```python
from build123d import *


with BuildPart() as part:
    # Sketch1 → Revolve2 (revolve)
    with BuildSketch(Plane.XY):
        with BuildLine():
            Line((-50.8, 69.85), (-50.8, 82.55))
            Line((-50.8, 82.55), (101.6, 82.55))
            Line((101.6, 82.55), (101.6, 12.7))
            Line((101.6, 12.7), (0, 12.7))
            Line((0, 12.7), (0, 25.4))
            ThreePointArc((0, 25.4), (-2.025659238, 31.58997261), (-7.62, 34.925))
            Line((-7.62, 34.925), (-24.13, 34.925))
            ThreePointArc((-24.13, 34.925), (-29.664711714, 38.307730629), (-31.75, 44.45))
            Line((-31.75, 44.45), (-31.75, 57.15))
            ThreePointArc((-31.75, 57.15), (-35.469743879, 66.130256121), (-44.45, 69.85))
            Line((-44.45, 69.85), (-50.8, 69.85))
        make_face()
    revolve(axis=Axis((0, 0, 0), (1, 0, 0)))


solid = part.part
```
The model under review builds one solid part; all positions refer to its coordinate system, in mm. A direction names the side the tool comes from. Round coordinates to 2 decimals unless told otherwise and drop trailing zeros. Loops run counter-clockwise (first coordinate to the right, second up) from the corner with the lowest first, then second, coordinate; pieces in that order, holes last. Notation, with made-up numbers: (-32.5, 9) -> (20.5, 9) arc R24 cw to (20.5, 47) -> close; hole circle Ø2 at (33, -19.75). An arc over 180 degrees is marked (long way). Answer as a JSON object with one key per item and string values. Group by question number.
1) Mouldability with a two-part tool opening along Y and no side actions: class faces 1 (the face through (26.467, -17.895, -80.587)), 2 (the face through (-47.669, -55.431, -42.503)), 3 (the face through (101.6, -1, -17)) as released by +Y, released by -Y, zero draft, split by the parting line, or undercut.
2) For pin 1 Ø5 at (x, y) = (60, -28.5) entering from -Z; pin 2 Ø4 at (x, z) = (26, -32) entering from -Y; pin 3 Ø3 at (y, z) = (63, 1.5) entering from -X; pin 4 Ø15 at (y, z) = (0, 0) entering from +X, all flat-tipped, find the tip position at first contact; note any pin that passes through.
3) We need section C-C on x = 18.5. Write out the cut boundary in (y, z), then the cut area to 3 significant figures.
4) For line 1 (Z direction, x = 60, y = 0); line 2 (Z direction, x = -47, y = 0); line 3 (X direction, y = 15, z = -10.5), list the stretches that pass through material, from the lowest coordinate up. Write a range as [from, to].
5) We need section A-A on z = 0. Write out the cut boundary in (x, y) (3 decimals), then the cut area to 3 significant figures.
6) For faces 4 (the face through (0, -5, 12)), 5 (the face through (50.09, -2.75, -12.4)), list the 3-axis set-ups (+Z, -Z, +X, -X, +Y, -Y) from which the entire face can be reached by the end or side of a thin tool; tool diameter is ignored.
7) We need section D-D on x = -39.5. Write out the cut boundary in (y, z), then the cut area to 3 significant figures.
Result set:
{
 "1": {"face 1": "split by the parting line", "face 2": "undercut", "face 3": "zero draft"},
 "2": {"pin 1": "z = -78.35", "pin 2": "y = -76.91", "pin 3": "x = -34.11", "pin 4": "through"},
 "3": {"outline": "circle Ø165.1 at (0, 0); hole circle Ø25.4 at (0, 0)", "area": "20,900 mm²"},
 "4": {"line 1": "[-82.55, -12.7], [12.7, 82.55]", "line 2": "[-82.55, -69.85], [69.85, 82.55]", "line 3": "[0, 101.6]"},
 "5": {"outline": "(-50.8, -82.55) -> (101.6, -82.55) -> (101.6, -12.7) -> (0, -12.7) -> (0, -25.4) arc R9.282 cw to (-7.62, -34.925) -> (-24.13, -34.925) arc R9.525 ccw to (-31.75, -44.45) -> (-31.75, -57.15) arc R12.7 cw to (-44.45, -69.85) -> (-50.8, -69.85) -> close; (-50.8, 69.85) -> (-44.45, 69.85) arc R12.7 cw to (-31.75, 57.15) -> (-31.75, 44.45) arc R9.525 ccw to (-24.13, 34.925) -> (-7.62, 34.925) arc R9.282 cw to (0, 25.4) -> (0, 12.7) -> (101.6, 12.7) -> (101.6, 82.55) -> (-50.8, 82.55) -> close", "area": "17,800 mm²"},
 "6": {"face 4": "-X", "face 5": "+X, -X"},
 "7": {"outline": "circle Ø165.1 at (0, 0); hole circle Ø137.69 at (0, 0)", "area": "6,520 mm²"}
}
